For this review, take the finished solid that the model builds, in its own axes (mm). A direction names the side the tool comes from. Coordinates: 2 decimals unless noted, no trailing zeros. Write each loop counter-clockwise with the first axis right and the second up, starting at its lowest first coordinate (ties: lowest second). Pieces come first, ordered by that corner, then holes. Notation, with made-up numbers: (-23, -32) - (24, -32) arc R21 ccw to (24, -4) - close; hole circle Ø10 at (31.25, -24). An arc over 180 degrees is marked (long way). Write each question's results on one line, items separated by ' | '.
from build123d import *

# Parameters (mm, degrees)
F0_W          = 2.54
F0_H          = 12.7
F3_DEPTH      = 25.4
F2_R          = 69.85
F4_DEPTH      = 25.4
F4_DEPTH_BACK = 25.4


with BuildPart() as f1:
    # F0 (on Front) → F1 (revolve)
    with BuildSketch(Plane.XZ):
        with Locations((-15.5575, 6.35)):
            Rectangle(F0_W, F0_H)
        Polygon((-16.8275, 12.7), (-14.2875, 12.7), (-14.2875, 15.24), (-20.6375, 15.24), (-20.6375, 12.7), align=None)
    revolve(axis=Axis((0, 0, 10.8147247049), (0, 0, 1)))

    # F3 (add): a face of the model
    f3_faces = [f1.faces().sort_by_distance(p)[0] for p in [
        (16.3515464256, 0, 0),
    ]]
    extrude(f3_faces, amount=F3_DEPTH)

    # F2 (on Front) → F4 (cut, two sides)
    with BuildSketch(Plane.XZ) as f4_sk:
        with Locations((0, -69.85)):
            Circle(F2_R)
    extrude(amount=-F4_DEPTH, mode=Mode.SUBTRACT)
    extrude(f4_sk.sketch, amount=F4_DEPTH_BACK, mode=Mode.SUBTRACT)


solid = f1.part
Q1. Wall thickness on line 1 along Y through (x, z) = (-0.5, 11); line 2 along X through (y, z) = (0, 7); line 3 along Z through (x, y) = (18.5, -9): over which ranges is each line inside the solid? List them lowest first. Write a range as from..to.
Results found:
line 1: -16.82..-14.28, 14.28..16.82 | line 2: -16.83..-14.29, 14.29..16.83 | line 3: 12.7..15.24
Q2. Take a section at A-A on y = 0. State the section outline as (x, z) points.
Results found:
outline: (-20.64, 12.7) - (-16.83, 12.7) - (-16.83, -2.06) arc R69.85 cw to (-14.29, -1.48) - (-14.29, 15.24) - (-20.64, 15.24) - close; (14.29, -1.48) arc R69.85 cw to (16.83, -2.06) - (16.83, 12.7) - (20.64, 12.7) - (20.64, 15.24) - (14.29, 15.24) - close
Q3. For pin 1 (1.5 mm diameter, centred on x = -2, y = 12, fed in from -Z); pin 2 (1 mm diameter, centred on y = -14, z = 9, fed in from +X); pin 3 (3 mm diameter, centred on x = -8, z = 11.5, fed in from -Y); pin 4 (8 mm diameter, centred on x = 14.5, z = 2, fed in from +Y), all flat-tipped, find the tip position at first contact; note any pin that passes through.
Results found:
pin 1: through | pin 2: x = 10.05 | pin 3: y = -19.38 | pin 4: y = 13.15
Q4. Mouldability with a two-part tool opening along X and no side actions: class faces 1 (the face through (17, 0, 12.7)), 2 (the face through (5.115, 13.636, -0.188)), 3 (the face through (4.474, 20.147, 13.952)) as pulls with the +X half, pulls with the -X half, needs draft (parallel to the pull), parting line crosses it, or undercut.
Results found:
face 1: needs draft | face 2: undercut | face 3: parting line crosses it
Q5. Take a section at D-D on x = -15.5. State the section outline as (y, z) points.
Results found:
outline: (-13.63, 12.7) - (-6.55, 12.7) - (-6.55, -1.74) - (6.55, -1.74) - (6.55, 12.7) - (13.63, 12.7) - (13.63, 15.24) - (-13.63, 15.24) - close
Q6. Take a section at C-C on z = 10.5. State the section outline as (x, y) points (1 decimal), plus the area to 3 significant figures.
Results found:
outline: circle Ø33.7 at (0, 0); hole circle Ø28.6 at (0, 0) | area: 248 mm2
Q7. For faces 4 (the face through (3.648, 16.427, 5.424)), 5 (the face through (14.274, -0.628, 6.998)), list the 3-axis set-ups (+Z, -Z, +X, -X, +Y, -Y) from which the entire face can be reached by the end or side of a thin tool; tool diameter is ignored.
Results found:
face 4: -Z | face 5: +Z, -Z
Q8. Take a section at B-B on x = 0. State the section outline as (y, z) points, plus the area to 3 significant figures.
Results found:
outline: (-20.64, 12.7) - (-16.83, 12.7) - (-16.83, 0) - (-14.29, 0) - (-14.29, 15.24) - (-20.64, 15.24) - close; (14.29, 0) - (16.83, 0) - (16.83, 12.7) - (20.64, 12.7) - (20.64, 15.24) - (14.29, 15.24) - close | area: 96.8 mm2
